```python
from build123d import *

# Parameters (mm, degrees)
F1_DEPTH = 76.5
F3_DEPTH = 66
F4_R     = 2.5
F5_DEPTH = 5.501


with BuildPart() as f1:
    # F0 (on Top) → F1 (new body)
    with BuildSketch(Plane.XY):
        Polygon((18.557011, -19.5), (16.375, 0), (0, 0), (-16.375, 0), (-18.557011, -19.5), (-26.757011, -19.5), (-26.757011, -25), (-11.122521, -25), (-9.5, -10.5), (0, -10.5), (9.5, -10.5), (11.122521, -25), (26.757011, -25), (26.757011, -19.5), align=None)
    extrude(amount=F1_DEPTH)

    # F2 (on face) → F3 (cut)
    with BuildSketch(Plane.XY.offset(76.5)):
        Polygon((9.6, 0), (-9.6, 0), (-9.6, -3.5), (-12.9, -3.5), (-12.9, -7), (12.9, -7), (12.9, -3.5), (9.6, -3.5), align=None)
    extrude(amount=-F3_DEPTH, mode=Mode.SUBTRACT)

    # F4 (on face) → F5 (cut, through all)
    with BuildSketch(Plane(origin=(0, -19.5, 0), x_dir=(-1, 0, 0), z_dir=(0, 1, 0))):
        with Locations((22.657011, 10)):
            Circle(F4_R)
        with Locations((22.657011, 66.5)):
            Circle(F4_R)
        with Locations((-22.657011, 10)):
            Circle(F4_R)
        with Locations((-22.657011, 66.5)):
            Circle(F4_R)
    extrude(amount=-F5_DEPTH, mode=Mode.SUBTRACT)


solid = f1.part
```
Could you check a few things on this model? Use its own coordinates, in mm. A direction names the side the tool comes from. Round coordinates to 2 decimals unless told otherwise and drop trailing zeros. Write each loop counter-clockwise with the first axis right and the second up, starting at its lowest first coordinate (ties: lowest second). Pieces come first, ordered by that corner, then holes.
(1) Suppose I cut it at C-C on x = -21. Write out the boundary of the cut face in (y, z), and give its area (3 significant figures).
Findings below:
outline: (-25, 0) - (-19.5, 0) - (-19.5, 8.13) - (-25, 8.13) - close; (-25, 11.87) - (-19.5, 11.87) - (-19.5, 64.63) - (-25, 64.63) - close; (-25, 68.37) - (-19.5, 68.37) - (-19.5, 76.5) - (-25, 76.5) - close
area: 380 mm2
(2) Suppose I cut it at B-B on y = -23. Write out the boundary of the cut face in (x, z).
Findings below:
outline: (-26.76, 0) - (-10.9, 0) - (-10.9, 76.5) - (-26.76, 76.5) - close; (10.9, 0) - (26.76, 0) - (26.76, 76.5) - (10.9, 76.5) - close; hole circle Ø5 at (-22.66, 10); hole circle Ø5 at (-22.66, 66.5); hole circle Ø5 at (22.66, 10); hole circle Ø5 at (22.66, 66.5)
(3) For pin 1 (8 mm diameter, centred on y = -8.5, z = 68, fed in from +X); pin 2 (9 mm diameter, centred on x = 24.5, z = 51, fed in from +Y); pin 3 (5.5 mm diameter, centred on x = -4.5, y = -2.5, fed in from +Z), each with a flat end and sliding along its axis, tell me the tip position at first contact or that it passes through.
Findings below:
pin 1: stops at x = 17.77
pin 2: stops at y = -19.5
pin 3: stops at z = 10.5
(4) Suppose I cut it at D-D on z = 6. Write out the boundary of the cut face in (x, y) (3 decimals).
Findings below:
outline: (-26.757, -25) - (-11.123, -25) - (-9.5, -10.5) - (9.5, -10.5) - (11.123, -25) - (26.757, -25) - (26.757, -19.5) - (18.557, -19.5) - (16.375, 0) - (-16.375, 0) - (-18.557, -19.5) - (-26.757, -19.5) - close
(5) Which directions (+Z, -Z, +X, -X, +Y, -Y) give clear straight access to the entire face, cutting with the end or side of a thin tool? Please do faces 4 (the face through (-23, -19.5, 38)), 5 (the face through (23, -19.5, 38)), 6 (the face through (12.9, -5, 44)).
Findings below:
face 4: +Z, -Z, -X, +Y
face 5: +Z, -Z, +X, +Y
face 6: +Z
(6) Thinking about a two-plate mould opening in Z: for faces 1 (the face through (24.64, -22.21, 64.98)), 2 (the face through (-2, -9, 76.5)), 3 (the face through (-10.323, -17.851, 37.714)), which applies, +Z half, -Z half, draft (parallel to the pull), parting line (faces both ways), or undercut?
Findings below:
face 1: undercut
face 2: +Z half
face 3: draft
(7) Suppose I cut it at A-A on z = 66.5. Write out the boundary of the cut face in (x, y) (3 decimals).
Findings below:
outline: (-26.757, -25) - (-25.157, -25) - (-25.157, -19.5) - (-26.757, -19.5) - close; (-20.157, -25) - (-11.123, -25) - (-9.5, -10.5) - (9.5, -10.5) - (11.123, -25) - (20.157, -25) - (20.157, -19.5) - (18.557, -19.5) - (16.375, 0) - (9.6, 0) - (9.6, -3.5) - (12.9, -3.5) - (12.9, -7) - (-12.9, -7) - (-12.9, -3.5) - (-9.6, -3.5) - (-9.6, 0) - (-16.375, 0) - (-18.557, -19.5) - (-20.157, -19.5) - close; (25.157, -25) - (26.757, -25) - (26.757, -19.5) - (25.157, -19.5) - close
(8) If I drill on probe 1 along Y at (x, z) = (3.5, 50); probe 2 along Y at (x, z) = (-19, 67); probe 3 along X at (y, z) = (-20.5, 70.5), over which ranges is the centre line in solid material (lowest first)?
Findings below:
probe 1: y = -10.5 to -7
probe 2: y = -25 to -19.5
probe 3: x = -26.76 to -10.62, 10.62 to 26.76
